from build123d import *

# Parameters (mm, degrees)
SKETCH1_R           = 3.5
SKETCH1_R_2         = 6.35
BOSS_EXTRUDE1_DEPTH = 89
SKETCH3_R           = 3.5
CUT_EXTRUDE2_DEPTH  = 8
SKETCH4_R           = 5
SKETCH4_R_2         = 3.5
BOSS_EXTRUDE2_DEPTH = 8
BOSS_EXTRUDE3_DEPTH = 7
SKETCH2_W           = 66.8
SKETCH2_H           = 348.711986474
CUT_EXTRUDE1_DEPTH  = 200
SKETCH8_W           = 74.8
SKETCH8_H           = 72.985639166
CUT_EXTRUDE3_DEPTH  = 7
SKETCH7_R           = 12.5
SKETCH7_W           = 109.075865198
SKETCH7_H           = 3
BOSS_EXTRUDE5_DEPTH = 66.8
SKETCH9_R           = 6.35
BOSS_EXTRUDE6_DEPTH = 3
SKETCH10_R          = 3.175
BOSS_EXTRUDE7_DEPTH = 66.8
CUT_EXTRUDE4_DEPTH  = 103


with BuildPart() as part:
    # Sketch1 → Boss-Extrude1 (new body)
    with BuildSketch(Plane.XY):
        with BuildLine():
            Line((48.479853629, 174.820410959), (48.479853629, 88.320410959))
            Line((48.479853629, 88.320410959), (-33.747283956, -13.279329595))
            Line((-33.747283956, -13.279329595), (-45.860496742, -20.29859423))
            Line((-45.860496742, -20.29859423), (-81.750845565, -64.644660941))
            Line((-81.750845565, -64.644660941), (-46.395506505, -100))
            Line((-46.395506505, -100), (72.579853629, -100))
            Line((72.579853629, -100), (72.579853629, 83.820410959))
            Line((72.579853629, 83.820410959), (67.579853629, 83.820410959))
            Line((67.579853629, 83.820410959), (67.579853629, 174.820410959))
            ThreePointArc((67.579853629, 174.820410959), (58.029853629, 184.370410959), (48.479853629, 174.820410959))
        make_face()
        Circle(SKETCH1_R, mode=Mode.SUBTRACT)
        with Locations((58.029853629, 138.320410959)):
            Circle(SKETCH1_R_2, mode=Mode.SUBTRACT)
        with Locations((58.029853629, 174.820410959)):
            Circle(SKETCH1_R_2, mode=Mode.SUBTRACT)
    extrude(amount=-BOSS_EXTRUDE1_DEPTH)

    # Sketch3 → Cut-Extrude2 (cut)
    with BuildSketch(Plane.XY):
        with BuildLine():
            ThreePointArc((-70.750928369, -62.916656075), (-72.139270825, -59.798970454), (-71.085322214, -56.552949701))
            Line((-71.085322214, -56.552949701), (-44.298080789, -23.454670242))
            ThreePointArc((-44.298080789, -23.454670242), (-43.692467175, -22.832236636), (-42.983894314, -22.330125149))
            Line((-42.983894314, -22.330125149), (-31.631604371, -15.751793807))
            Line((-31.631604371, -15.751793807), (37.252005086, 69.360701347))
            ThreePointArc((37.252005086, 69.360701347), (50.583965109, 73.123701006), (58.579853629, 61.811446975))
            Line((58.579853629, 61.811446975), (58.579853629, -92.0375))
            ThreePointArc((58.579853629, -92.0375), (57.184949674, -95.405096045), (53.817353629, -96.8))
            Line((53.817353629, -96.8), (-34.894892353, -96.8))
            ThreePointArc((-34.894892353, -96.8), (-36.7174222, -96.437476274), (-38.262488399, -95.405096045))
            Line((-38.262488399, -95.405096045), (-70.750928369, -62.916656075))
        make_face()
        Circle(SKETCH3_R, mode=Mode.SUBTRACT)
        with BuildLine():
            ThreePointArc((51.479853629, 126.145410959), (52.409789598, 128.390474989), (54.654853629, 129.320410959))
            Line((54.654853629, 129.320410959), (61.404853629, 129.320410959))
            ThreePointArc((61.404853629, 129.320410959), (63.649917659, 128.390474989), (64.579853629, 126.145410959))
            Line((64.579853629, 126.145410959), (64.579853629, 85.495410959))
            ThreePointArc((64.579853629, 85.495410959), (63.649917659, 83.250346929), (61.404853629, 82.320410959))
            Line((61.404853629, 82.320410959), (54.654853629, 82.320410959))
            ThreePointArc((54.654853629, 82.320410959), (52.409789598, 83.250346929), (51.479853629, 85.495410959))
            Line((51.479853629, 85.495410959), (51.479853629, 126.145410959))
        make_face()
        with BuildLine():
            ThreePointArc((51.479853629, 162.645410959), (52.409789598, 164.890474989), (54.654853629, 165.820410959))
            Line((54.654853629, 165.820410959), (61.404853629, 165.820410959))
            ThreePointArc((61.404853629, 165.820410959), (63.649917659, 164.890474989), (64.579853629, 162.645410959))
            Line((64.579853629, 162.645410959), (64.579853629, 150.495410959))
            ThreePointArc((64.579853629, 150.495410959), (63.649917659, 148.250346929), (61.404853629, 147.320410959))
            Line((61.404853629, 147.320410959), (54.654853629, 147.320410959))
            ThreePointArc((54.654853629, 147.320410959), (52.409789598, 148.250346929), (51.479853629, 150.495410959))
            Line((51.479853629, 150.495410959), (51.479853629, 162.645410959))
        make_face()
    cut_extrude2 = extrude(amount=-CUT_EXTRUDE2_DEPTH, mode=Mode.SUBTRACT)

    # Sketch4 → Boss-Extrude2 (add)
    with BuildSketch(Plane.XY.offset(-8)):
        Circle(SKETCH4_R)
        Circle(SKETCH4_R_2, mode=Mode.SUBTRACT)
    extrude(amount=BOSS_EXTRUDE2_DEPTH)

    # Sketch5 → Boss-Extrude3 (add)
    with BuildSketch(Plane.XY):
        with BuildLine():
            Line((58.579853629, 61.811446975), (58.579853629, -92.0375))
            Line((58.579853629, -92.0375), (58.579853629, -100))
            Line((58.579853629, -100), (65.579853629, -100))
            Line((65.579853629, -100), (65.579853629, 74.645410959))
            ThreePointArc((65.579853629, 74.645410959), (66.509789598, 76.890474989), (68.754853629, 77.820410959))
            Line((68.754853629, 77.820410959), (72.579853629, 77.820410959))
            Line((72.579853629, 77.820410959), (72.579853629, 80.320410959))
            Line((72.579853629, 80.320410959), (58.579853629, 80.320410959))
            Line((58.579853629, 80.320410959), (58.579853629, 61.811446975))
        make_face()
    boss_extrude3 = extrude(amount=BOSS_EXTRUDE3_DEPTH)

    # Mirror2: Cut-Extrude2, Boss-Extrude3 across plane
    add(cut_extrude2.mirror(Plane.XY.offset(-44.5)), mode=Mode.SUBTRACT)
    add(boss_extrude3.mirror(Plane.XY.offset(-44.5)))

    # Sketch2 → Cut-Extrude1 (cut)
    with BuildSketch(Plane(origin=(72.579853629, 0, 0), x_dir=(0, 0, -1), z_dir=(1, 0, 0))):
        with Locations((44.5, 44.534818405)):
            Rectangle(SKETCH2_W, SKETCH2_H)
    extrude(amount=-CUT_EXTRUDE1_DEPTH, mode=Mode.SUBTRACT)

    # Sketch8 → Cut-Extrude3 (cut)
    with BuildSketch(Plane(origin=(-73.197753253, -73.197753253, 0), x_dir=(0, 0, 1), z_dir=(-0.707106781, -0.707106781, 0))):
        with Locations((-44.5, -19.729026559)):
            Rectangle(SKETCH8_W, SKETCH8_H)
    extrude(amount=-CUT_EXTRUDE3_DEPTH, mode=Mode.SUBTRACT)

    # Sketch7 → Boss-Extrude5 (add)
    with BuildSketch(Plane.XY.offset(-77.9)):
        Polygon((46.479853629, 31.730850002), (46.479853629, 33.320410959), (6.661618145, -15.878947224), (4.279039025, -13.950668076), (-38.39575734, -66.679589041), (18.545061094, -66.679589041), (46.479853629, -66.679589041), (46.479853629, -65.679589041), (6.815381875, -65.679589041), (-36.299962765, -65.679589041), (4.427255206, -15.357093319), (6.809834326, -17.285372467), align=None)
        Polygon((53.479853629, -66.679589041), (53.479853629, 33.320410959), (46.479853629, 33.320410959), (46.479853629, 31.730850002), (46.479853629, -65.679589041), (46.479853629, -66.679589041), align=None)
        with Locations((35, -82)):
            Circle(SKETCH7_R)
        with Locations((0, -82)):
            Circle(SKETCH7_R)
        with Locations((18.04192103, -98.5)):
            Rectangle(SKETCH7_W, SKETCH7_H)
    extrude(amount=BOSS_EXTRUDE5_DEPTH)

    # Sketch9 → Boss-Extrude6 (add)
    with BuildSketch(Plane(origin=(0, 0, -11.1), x_dir=(-1, 0, 0), z_dir=(0, 0, -1))):
        with Locations((-58.029853629, 174.820410959)):
            Circle(SKETCH9_R)
    boss_extrude6 = extrude(amount=-BOSS_EXTRUDE6_DEPTH)

    # Mirror3: Boss-Extrude6 across plane
    add(boss_extrude6.mirror(Plane.XY.offset(-44.5)))

    # Sketch10 → Boss-Extrude7 (add)
    with BuildSketch(Plane(origin=(0, 0, -11.1), x_dir=(-1, 0, 0), z_dir=(0, 0, -1))):
        with Locations((-58.029853629, 174.820410959)):
            Circle(SKETCH10_R)
    extrude(amount=BOSS_EXTRUDE7_DEPTH)

    # Sketch11 → Cut-Extrude4 (cut)
    with BuildSketch(Plane.XY.offset(7)):
        Polygon((62.079853629, -100), (72.579853629, -85), (72.579853629, -100), align=None)
    extrude(amount=-CUT_EXTRUDE4_DEPTH, mode=Mode.SUBTRACT)


solid = part.part
Geometry check sheet. Reference: the model listing, model coordinates, mm. A direction names the side the tool comes from. Coordinates: 2 decimals unless noted, no trailing zeros. Order: outer loops, then holes, each group sorted by start corner. A loop starts at its lowest first (then second) coordinate and runs counter-clockwise, first axis right, second up. Notation, with made-up numbers: (56, -21.75) - (65, -21.75) arc R18 cw to (65, -1.75) - close; hole circle Ø7 at (64.25, 42). An arc over 180 degrees is marked (long way). One line per item, written item: value.
(1) Thickness scan on probe 1 along Y at (x, z) = (51, -18.5); probe 2 along Z at (x, y) = (-57.5, -58); probe 3 along Z at (x, y) = (-63, -81.5). Record the ranges inside material, lowest first. Write a range as from..to.
Data:
probe 1: y = -100..-97, -66.68..33.32
probe 2: z = -81..-77.9, -11.1..-8
probe 3: z = -89..-81.9, -7.1..0
(2) Release check for a two-part mould opening along X. For faces 6 (the face through (-39.72, -16.74, -83.37)), 7 (the face through (-54.28, -79.39, -3.94)), 8 (the face through (58.24, 184.37, -83.37)) record: +X half, -X half, draft (parallel to the pull), parting line (faces both ways), or undercut.
Data:
face 6: -X half
face 7: undercut
face 8: parting line
(3) Depth check by flat-ended pin: pin 1 Ø9 at (y, z) = (155, -5) entering from +X; pin 2 Ø16.5 at (y, z) = (8, -1.5) entering from -X; pin 3 Ø2.5 at (x, z) = (12.5, -3) entering from +Y. Enter the tip coordinate at first touch or a pass-through.
Data:
pin 1: stops at x = 67.58
pin 2: stops at x = -23.2
pin 3: stops at y = 45.41
(4) Access from +Z, -Z, +X, -X, +Y, -Y to the whole of each face (thin tool, end or side, straight path). Record for faces 1 (the face through (-72.136, -59.848, -85.056)), 2 (the face through (-1.627, -69.606, -44.968)), 3 (the face through (69, -7, 0)), 4 (the face through (48.48, 132, -5)), 5 (the face through (-59, -82, -7.1)).
Data:
face 1: -Z
face 2: none
face 3: +Z, +X, -Y
face 4: +Z, -Z, -X, +Y
face 5: -X, -Y
(5) Sectioned sample at B-B (x = -68). Enter the section's corners in (y, z).
Data:
outline: (-78.4, -89) - (-65.67, -89) - (-65.67, -81) - (-52.74, -81) - (-52.74, -89) - (-47.65, -89) - (-47.65, -77.9) - (-68.5, -77.9) - (-68.5, -81.9) - (-78.4, -81.9) - close; (-78.4, -7.1) - (-68.5, -7.1) - (-68.5, -11.1) - (-47.65, -11.1) - (-47.65, 0) - (-52.74, 0) - (-52.74, -8) - (-65.67, -8) - (-65.67, 0) - (-78.4, 0) - close
(6) Sectioned sample at D-D (x = 34). Enter the section's corners in (y, z), and give its area (3 significant figures).
Data:
outline: (-100, -89) - (-96.8, -89) - (-96.8, -81) - (65.34, -81) - (65.34, -89) - (70.43, -89) - (70.43, -77.9) - (17.9, -77.9) - (17.9, -11.1) - (70.43, -11.1) - (70.43, 0) - (65.34, 0) - (65.34, -8) - (-96.8, -8) - (-96.8, 0) - (-100, 0) - close; hole (-97, -77.9) - (-94.46, -77.9) - (-94.46, -11.1) - (-97, -11.1) - close; hole (-69.54, -77.9) - (-66.68, -77.9) - (-66.68, -11.1) - (-69.54, -11.1) - close; hole (-65.68, -77.9) - (16.31, -77.9) - (16.31, -11.1) - (-65.68, -11.1) - close
area: 3,230 mm^2
(7) Sectioned sample at C-C (y = 58). Enter the section's corners in (x, z).
Data:
outline: (23.94, -89) - (28.06, -89) - (28.06, -81) - (58.58, -81) - (58.58, -96) - (65.58, -96) - (65.58, -89) - (72.58, -89) - (72.58, -77.9) - (23.94, -77.9) - close; (23.94, -11.1) - (72.58, -11.1) - (72.58, 0) - (65.58, 0) - (65.58, 7) - (58.58, 7) - (58.58, -8) - (28.06, -8) - (28.06, 0) - (23.94, 0) - close
(8) Sectioned sample at A-A (z = -33.5). Enter the section's corners in (x, y) (3 decimals), and give its area (3 significant figures).
Data:
outline: (-38.396, -66.68) - (53.48, -66.68) - (53.48, 33.32) - (46.48, 33.32) - (6.662, -15.879) - (4.279, -13.951) - close; (-36.496, -100) - (62.08, -100) - (64.18, -97) - (-36.496, -97) - close; circle Ø25 at (0, -82); circle Ø25 at (35, -82); circle Ø6.35 at (58.03, 174.82); hole (-36.3, -65.68) - (46.48, -65.68) - (46.48, 31.731) - (6.81, -17.285) - (4.427, -15.357) - close
area: 2,230 mm^2
